Source: CAD feature listing. Evaluate the final solid. Frame: model axes, mm. Face numbers are marked on the shaded views. A direction names the side the tool comes from. Coordinates: 2 decimals unless noted, no trailing zeros. Loops run counter-clockwise (first coordinate to the right, second up) from the corner with the lowest first, then second, coordinate; pieces in that order, holes last.
Item 1: Reachability of the marked faces 1 and 2 from +Z, -Z, +X, -X, +Y, -Y: full face, straight path, thin tool, end or side. Return the list, or none.
Item 2: Line query: probe 1 along Y at (x, z) = (14, -2.5) (1 decimal); probe 2 along Z at (x, y) = (-25.4, 14.55); probe 3 along Z at (x, y) = (-25, -14). Output: solid intervals per line, ascending.
Item 3: Section query A-A, the plane z = 12.7. State how many separate pieces and enclosed holes the cut face has, then the cut area to 3 significant figures.
Item 4: Section query D-D, the plane x = -42. Return the cut outline in (y, z) (1 decimal), then the cut area to 3 significant figures.
Item 5: Pull-direction query (Y, two-part tool) for the marked faces 3, 4, 5 and 6; classes: +Y half, -Y half, draft (parallel to the pull), parting line (faces both ways), or undercut.
Item 6: Pin query (flat end, axial travel): pin 1 Ø21.5 at (x, y) = (-21, 1) entering from -Z; pin 2 Ø12 at (x, y) = (-38.5, 11) entering from -Z; pin 3 Ø6.5 at (x, z) = (-25.4, 12.7) entering from +Y; pin 4 Ø10 at (x, z) = (44.5, 6) entering from +Y. Return the tip coordinate at first contact, or that it passes through.
Item 7: Section query C-C, the plane y = 0. Return the cut outline in (x, z) (1 decimal), then the cut area to 3 significant figures.
```python
from build123d import *

# Parameters (mm, degrees)
F1_DEPTH       = 25.4
F3_DEPTH       = 4.7625
F5_D           = 7.9375
F5_DEPTH       = 12.7
F5_CSINK_D     = 12.7
F5_CSINK_ANGLE = 82
F5_TIP         = 2.3846655818
F6_R           = 2.54
F8_DEPTH       = 10.16
F9_T4_DEPTH    = 169.4252160848
F9_T9_DEPTH    = 169.4252160848


# Not quite as in the source:
# - a fillet or chamfer that OpenCascade refuses, or shapes differently, is made with other operations: its cross-section is extruded or revolved along the edge and cut away or added
# - a pattern or mirror of a feature is missing from the dataset's text; its kind, count and spacing are read off the source's solid
# - a feature names something its author has since deleted; it is built from what else it names


with BuildPart() as f1:
    # F0 (on Top) → F1 (new body)
    with BuildSketch(Plane.XY):
        with BuildLine():
            Line((38.1, 18.0975), (-50.8, 18.0975))
            Line((-50.8, 18.0975), (-50.8, 13.335))
            Line((-50.8, 13.335), (38.1, 13.335))
            ThreePointArc((38.1, 13.335), (51.435, 0), (38.1, -13.335))
            Line((38.1, -13.335), (-50.8, -13.335))
            Line((-50.8, -13.335), (-50.8, -18.0975))
            Line((-50.8, -18.0975), (38.1, -18.0975))
            ThreePointArc((38.1, -18.0975), (56.1975, 0), (38.1, 18.0975))
        make_face()
    extrude(amount=F1_DEPTH)

    # F2 (on face) → F3 (join)
    with BuildSketch(Plane.XY.offset(25.4)):
        with BuildLine():
            Line((38.1, 13.335), (-50.8, 13.335))
            Line((-50.8, 13.335), (-50.8, -13.335))
            Line((-50.8, -13.335), (38.1, -13.335))
            ThreePointArc((38.1, -13.335), (51.435, 0), (38.1, 13.335))
        make_face()
        with BuildLine():
            Line((38.1, 18.0975), (-50.8, 18.0975))
            Line((-50.8, 18.0975), (-50.8, 13.335))
            Line((-50.8, 13.335), (38.1, 13.335))
            ThreePointArc((38.1, 13.335), (51.435, 0), (38.1, -13.335))
            Line((38.1, -13.335), (-50.8, -13.335))
            Line((-50.8, -13.335), (-50.8, -18.0975))
            Line((-50.8, -18.0975), (38.1, -18.0975))
            ThreePointArc((38.1, -18.0975), (56.1975, 0), (38.1, 18.0975))
        make_face()
    extrude(amount=F3_DEPTH)

    # F5
    with Locations(Plane.XZ.offset(18.0975)):
        with Locations((-25.4, 12.7)):
            f5 = CounterSinkHole(F5_D / 2, F5_CSINK_D / 2, depth=F5_DEPTH, counter_sink_angle=F5_CSINK_ANGLE)
            with Locations((0, 0, -(F5_DEPTH + F5_TIP / 2))):  # 118° drill point
                Cone(0, F5_D / 2, F5_TIP, mode=Mode.SUBTRACT)

    # F5_copies: F5 across plane
    add(f5.mirror(Plane.ZX), mode=Mode.SUBTRACT)

    # F6
    f6_edges = [f1.edges().sort_by_distance(p)[0] for p in [
        (-50.8, 0, 30.1625),
        (-6.35, 18.0975, 30.1625),
        (-50.8, 18.0975, 15.08125),
        (56.1975, 0, 30.1625),
        (-6.35, -18.0975, 30.1625),
        (-50.8, -18.0975, 15.08125),
    ]]
    fillet(f6_edges, radius=F6_R)

    # F7 (on face) → F8 (join)
    with BuildSketch(Plane(origin=(0, 0, 0), x_dir=(1, 0, 0), z_dir=(0, 0, -1))):
        with BuildLine():
            ThreePointArc((38.1, -18.0975), (56.1975, 0), (38.1, 18.0975))
            Line((38.1, 18.0975), (0, 18.0975))
            Line((0, 18.0975), (0, 13.335))
            Line((0, 13.335), (38.1, 13.335))
            ThreePointArc((38.1, 13.335), (51.435, 0), (38.1, -13.335))
            Line((38.1, -13.335), (0, -13.335))
            Line((0, -13.335), (0, -18.0975))
            Line((0, -18.0975), (38.1, -18.0975))
        make_face()
    extrude(amount=F8_DEPTH)

    # F9: chamfer of 31.75 x 12.7 on 2 edges, made by hand


with BuildPart() as f9_tool2:
    # F9_s3 → F9_t4 (new body)
    with BuildSketch(Plane.XZ.offset(68.9963580424)):
        Polygon((31.75, -10.16), (0, 2.54), (0, -10.16), align=None)
    extrude(amount=-F9_T4_DEPTH)

    split(bisect_by=Plane.XY, keep=Keep.BOTTOM)


with BuildPart() as f1_1:
    add(f1.part)

    # F9_t1: cut F9_tool2
    add(f9_tool2.part, mode=Mode.SUBTRACT)


with BuildPart() as f9_tool7:
    # F9_s8 → F9_t9 (new body)
    with BuildSketch(Plane.XZ.offset(100.4288580424)):
        Polygon((0, 2.54), (31.75, -10.16), (0, -10.16), align=None)
    extrude(amount=-F9_T9_DEPTH)

    split(bisect_by=Plane.XY, keep=Keep.BOTTOM)


with BuildPart() as f1_2:
    add(f1_1.part)

    # F9_t6: cut F9_tool7
    add(f9_tool7.part, mode=Mode.SUBTRACT)


solid = f1_2.part
```
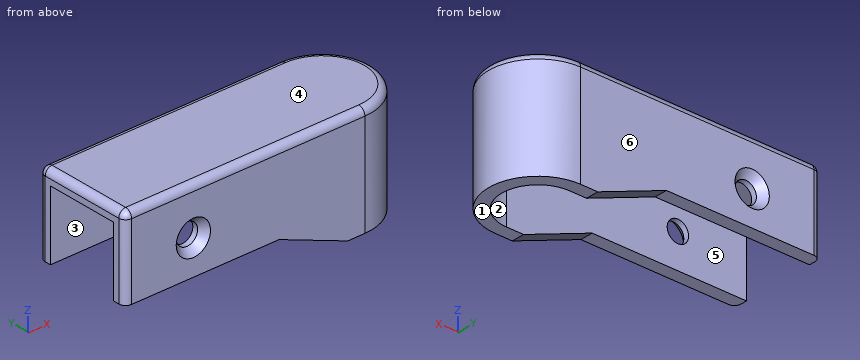
Verdict:
1. face 1: -Z, +X, -X, +Y, -Y
1. face 2: -Z, -X
2. probe 1: y = -18.1 to -13.3, 13.3 to 18.1
2. probe 2: z = 0 to 8.73, 16.67 to 30.16
2. probe 3: z = 0 to 8.75, 16.65 to 30.16
3. separate pieces: 3
3. enclosed holes: 0
3. area: 990 mm2
4. outline: (-18.1, 0) - (-13.3, 0) - (-13.3, 25.4) - (13.3, 25.4) - (13.3, 0) - (18.1, 0) - (18.1, 27.6) arc R2.5 ccw to (15.6, 30.2) - (-15.6, 30.2) arc R2.5 ccw to (-18.1, 27.6) - close
4. area: 412 mm2
5. face 3: undercut
5. face 4: draft
5. face 5: undercut
5. face 6: +Y half
6. pin 1: stops at z = 25.4
6. pin 2: stops at z = 0
6. pin 3: passes through
6. pin 4: stops at y = 18.04
7. outline: (-50.8, 25.4) - (51.4, 25.4) - (51.4, -10.2) - (56.2, -10.2) - (56.2, 27.6) arc R2.5 ccw to (53.7, 30.2) - (-48.3, 30.2) arc R2.5 ccw to (-50.8, 27.6) - close
7. area: 676 mm2
